For this review, take the finished solid that the model builds, in its own axes (mm). A direction names the side the tool comes from. Round coordinates to 2 decimals unless told otherwise and drop trailing zeros. Order: outer loops, then holes, each group sorted by start corner. A loop starts at its lowest first (then second) coordinate and runs counter-clockwise, first axis right, second up. Notation, with made-up numbers: M -13.5,4.25 L 34.5,4.25 A23 cw 34.5,41.25 Z; hole C -17.5,4 d5. An arc over 180 degrees is marked long. Answer as a JSON object with one key per item and string values.
from build123d import *

# Parameters (mm, degrees)
EXTRUDE_1_DEPTH             = 9
CUT_EXTRUDE_1_DEPTH         = 21.518284529
HOLE_WIZARD_M2_2_AT_2_COUNT = 2
HOLE_WIZARD_M2_2_AT_2_PITCH = 6
HOLE_WIZARD_M2_2_AT_3_COUNT = 2
HOLE_WIZARD_M2_2_AT_3_PITCH = 33
HOLE_WIZARD_M2_2_AT_4_COUNT = 2
HOLE_WIZARD_M2_2_AT_4_PITCH = 33.541019662
HOLE_WIZARD_M2_3_AT_2_COUNT = 2
HOLE_WIZARD_M2_3_AT_2_PITCH = 6.4
HOLE_WIZARD_M2_3_AT_3_COUNT = 2
HOLE_WIZARD_M2_3_AT_3_PITCH = 22.336517186
HOLE_WIZARD_M2_3_AT_4_COUNT = 2
HOLE_WIZARD_M2_3_AT_4_PITCH = 21.4


with BuildPart() as part:
    # 草图1 → 凸台-拉伸1 (new body)
    with BuildSketch(Plane.XY):
        Polygon((-12, 0), (12, 0), (14, 2), (14, 3), (18, 3), (18, 2), (15, 2), (15, 1.585786438), (12.414213562, -1), (-12.414213562, -1), (-15, 1.585786438), (-15, 2), (-18, 2), (-18, 3), (-14, 3), (-14, 2), align=None)
    extrude(amount=EXTRUDE_1_DEPTH)

    # 草图2 → 切除-拉伸1 (cut, through all)
    with BuildSketch(Plane.XZ.offset(1)):
        Polygon((-10.414213562, 9), (-8, 6), (8, 6), (10.414213562, 9), align=None)
    extrude(amount=-CUT_EXTRUDE_1_DEPTH, mode=Mode.SUBTRACT)

    # 草图7 → M2 螺纹孔2 (revolve, cut)
    with BuildSketch(Plane(origin=(-16.5, 2, 7.5), x_dir=(0, 0, -1), z_dir=(1, 0, 0))):
        Polygon((0, 0), (0, 1), (0.8, 1), (0.8, 0.225), (1.025, 0), align=None)
    hole_wizard_m2_2 = revolve(axis=Axis((-16.5, -4.35, 7.5), (0, 1, 0)), mode=Mode.SUBTRACT)

    # M2 螺纹孔2 at 2: M2 螺纹孔2 ×2
    with Locations(*[(0, 0, -i * HOLE_WIZARD_M2_2_AT_2_PITCH) for i in range(1, HOLE_WIZARD_M2_2_AT_2_COUNT)]):
        add(hole_wizard_m2_2, mode=Mode.SUBTRACT)

    # M2 螺纹孔2 at 3: M2 螺纹孔2 ×2
    with Locations(*[(i * HOLE_WIZARD_M2_2_AT_3_PITCH, 0, 0) for i in range(1, HOLE_WIZARD_M2_2_AT_3_COUNT)]):
        add(hole_wizard_m2_2, mode=Mode.SUBTRACT)

    # M2 螺纹孔2 at 4: M2 螺纹孔2 ×2
    with Locations(*[Vector(0.9838699100999075, 0, -0.17888543819998318) * (i * HOLE_WIZARD_M2_2_AT_4_PITCH) for i in range(1, HOLE_WIZARD_M2_2_AT_4_COUNT)]):
        add(hole_wizard_m2_2, mode=Mode.SUBTRACT)

    # 草图10 → M2 螺纹孔3 (revolve, cut)
    with BuildSketch(Plane(origin=(-10.7, -1, 7.7), x_dir=(0, 0, -1), z_dir=(1, 0, 0))):
        Polygon((0, 0), (0, 1), (0.8, 1), (0.8, 0.225), (1.025, 0), align=None)
    hole_wizard_m2_3 = revolve(axis=Axis((-10.7, -7.35, 7.7), (0, 1, 0)), mode=Mode.SUBTRACT)

    # M2 螺纹孔3 at 2: M2 螺纹孔3 ×2
    with Locations(*[(0, 0, -i * HOLE_WIZARD_M2_3_AT_2_PITCH) for i in range(1, HOLE_WIZARD_M2_3_AT_2_COUNT)]):
        add(hole_wizard_m2_3, mode=Mode.SUBTRACT)

    # M2 螺纹孔3 at 3: M2 螺纹孔3 ×2
    with Locations(*[Vector(0.9580723718836152, 0, -0.28652631682500634) * (i * HOLE_WIZARD_M2_3_AT_3_PITCH) for i in range(1, HOLE_WIZARD_M2_3_AT_3_COUNT)]):
        add(hole_wizard_m2_3, mode=Mode.SUBTRACT)

    # M2 螺纹孔3 at 4: M2 螺纹孔3 ×2
    with Locations(*[(i * HOLE_WIZARD_M2_3_AT_4_PITCH, 0, 0) for i in range(1, HOLE_WIZARD_M2_3_AT_4_COUNT)]):
        add(hole_wizard_m2_3, mode=Mode.SUBTRACT)


solid = part.part
1) Add section C-C on y = 0.5. State the section outline as (x, z) points.
Geometry check:
{"outline": "M -13.91,0 L -12.5,0 L -12.5,9 L -13.91,9 Z; M 12.5,0 L 13.91,0 L 13.91,9 L 12.5,9 Z"}
2) Machinability: for faces 1 (the flat face through (17, 2, 4)), 2 (the flat face through (13, 1, 4)), 3 (the cylindrical face through (11.19, -0.39, 1.93)), 4 (the flat face through (-16, 3, 4)), 5 (the flat face through (-0.1, -0.5, 6)), which of the approach directions +Z, -Z, +X, -X, +Y, -Y give a long, thin tool a straight path to every point of the face, cutting with its end or side? Answer none if there is none.
Geometry check:
{"face 1": "+Z, -Z, +X, -Y", "face 2": "+Z, -Z, +Y", "face 3": "+Y, -Y", "face 4": "+Z, -Z, +X, -X, +Y", "face 5": "+Z, +Y, -Y"}
3) For L1, parallel to X at y = 2.5, z = 7.5; L2, parallel to Z at x = 16.5, y = 2.5; L3, parallel to Z at x = -10.7, y = -0.35, list the stretches that pass through material, from the lowest coordinate up.
Geometry check:
{"L1": "x = -18 to -17.3, -15.7 to -14, 14 to 15.7, 17.3 to 18", "L2": "z = 0 to 0.7, 2.3 to 6.7, 8.3 to 9", "L3": "z = 0 to 0.5, 2.1 to 6.9, 8.5 to 9"}
4) Add section D-D on z = 1.3. State how many separate pieces and enclosed holes the cut face has, and give its area (3 significant figures).
Geometry check:
{"separate pieces": "5", "enclosed holes": "0", "area": "32.8 mm²"}
5) Insertion check: P1, Ø1.5, axis at x = 13.5, y = -0.5, coming from the +Z side; P2, Ø2.5, axis at x = -16.5, z = 6, coming from the -Y side; P3, Ø2, axis at x = 10.7, z = 7.7, coming from the -Y side (3 decimals); P4, Ø1, axis at x = 11, z = 2.5, coming from the +Y side. Each pin has a flat end and moves straight along its axis. Give the tip position at first contact, or say it passes through.
Geometry check:
{"P1": "stops at z = 9", "P2": "stops at y = 2", "P3": "stops at y = -0.975", "P4": "stops at y = 0"}
6) Add section B-B on z = 3. State the section outline as (x, y) points.
Geometry check:
{"outline": "M -18,2 L -15,2 L -15,1.59 L -12.41,-1 L 12.41,-1 L 15,1.59 L 15,2 L 18,2 L 18,3 L 14,3 L 14,2 L 12,0 L -12,0 L -14,2 L -14,3 L -18,3 Z"}
7) Mouldability with a two-part tool opening along X and no side actions: class faces 6 (the flat face through (0.1, -0.3, 0)), 7 (the cylindrical face through (-9.99, -0.39, 0.93)), 8 (the flat face through (18, 2.5, 4.4)) as +X half, -X half, draft (parallel to the pull), parting line (faces both ways), or undercut.
Geometry check:
{"face 6": "draft", "face 7": "undercut", "face 8": "+X half"}
8) Add section A-A on x = -16.5. State the section outline as (y, z) points (3 decimals), and give its area (3 significant figures).
Geometry check:
{"outline": "M 2,0 L 3,0 L 3,0.7 L 2.225,0.7 L 2,0.475 Z; M 2,2.525 L 2.225,2.3 L 3,2.3 L 3,6.7 L 2.225,6.7 L 2,6.475 Z; M 2,8.525 L 2.225,8.3 L 3,8.3 L 3,9 L 2,9 Z", "area": "5.70 mm²"}
